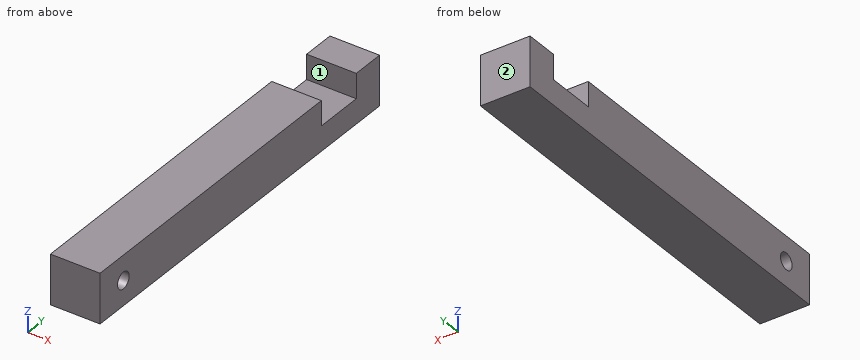
```python
from build123d import *

# Parameters (mm, degrees)
F0_W     = 19.05
F0_H     = 19.05
F1_DEPTH = 9.525
F0_H_2   = 120.65
F0_H_3   = 12.7
F2_DEPTH = 19.05
F4_D     = 6.35


with BuildPart() as f1:
    # F0 (on Top) → F1 (new body)
    with BuildSketch(Plane.XY):
        with Locations((-25.66231, 87.892967)):
            Rectangle(F0_W, F0_H)
    extrude(amount=F1_DEPTH)

    # F0 (on Top) → F2 (join)
    with BuildSketch(Plane.XY):
        with Locations((-25.66231, 18.042967)):
            Rectangle(F0_W, F0_H_2)
        with Locations((-25.66231, 103.767967)):
            Rectangle(F0_W, F0_H_3)
    extrude(amount=F2_DEPTH)

    # F4 (through all)
    with Locations(Plane(origin=(-35.18731, 0, 0), x_dir=(0, -1, 0), z_dir=(-1, 0, 0))):
        with Locations((29.582033, 9.525)):
            Hole(F4_D / 2)


solid = f1.part
```
Here's how the part is built. I have some questions about the finished solid (model axes, mm). Face numbers are marked on the shaded views. A direction names the side the tool comes from. Coordinates: 2 decimals unless noted, no trailing zeros. Order: outer loops, then holes, each group sorted by start corner. A loop starts at its lowest first (then second) coordinate and runs counter-clockwise, first axis right, second up.
1) Imagine slicing it at A-A on x = -32.5. List the corners of the cut face in (y, z) for me (3 decimals).
2) Imagine slicing it at B-B on z = 15.5. List the corners of the cut face in (x, y) for me, and give its area (3 significant figures).
3) Which directions (+Z, -Z, +X, -X, +Y, -Y) give clear straight access to the entire face, cutting with the end or side of a thin tool? Please do the marked faces 1 and 2.
4) I need wall thicknesses on line 1 (Y direction, x = -26.25, z = 14.5); line 2 (Z direction, x = -23, y = 80.5) (3 decimals); line 3 (Z direction, x = -31.5, y = -32). Which ranges of each line are inside material? Lowest first, please.
5) Imagine slicing it at C-C on y = 94.5. List the corners of the cut face in (x, z) for me (3 decimals), and give its area (3 significant figures).
6) Will this pin go through, and if not, where does the flat tip stop? pin 1 (4 mm diameter, centred on y = -29.58, z = 9.52, fed in from -X).
Response values:
1. outline: (-42.282, 0) - (110.118, 0) - (110.118, 19.05) - (97.418, 19.05) - (97.418, 9.525) - (78.368, 9.525) - (78.368, 19.05) - (-42.282, 19.05) - close; hole circle Ø6.35 at (-29.582, 9.525)
2. outline: (-35.19, -42.28) - (-16.14, -42.28) - (-16.14, 78.37) - (-35.19, 78.37) - close; (-35.19, 97.42) - (-16.14, 97.42) - (-16.14, 110.12) - (-35.19, 110.12) - close
2. area: 2,540 mm2
3. face 1: +Z, +X, -X
3. face 2: +Z, -Z, +X, -X, +Y
4. line 1: y = -42.28 to 78.37, 97.42 to 110.12
4. line 2: z = 0 to 9.525
4. line 3: z = 0 to 7.47, 11.58 to 19.05
5. outline: (-35.187, 0) - (-16.137, 0) - (-16.137, 9.525) - (-35.187, 9.525) - close
5. area: 181 mm2
6. pin 1: passes through
